Could you check a few things on this model? Use its own coordinates, in mm. Face numbers are marked on the shaded views. A direction names the side the tool comes from. Give positions to 0.01 mm unless a question says otherwise; leave off trailing zeros. Order: outer loops, then holes, each group sorted by start corner. A loop starts at its lowest first (then second) coordinate and runs counter-clockwise, first axis right, second up. Notation, with made-up numbers: (-28, 84) -> (-2, 84) arc R10 ccw to (-2, 88) -> close; hole circle Ø8 at (-13, -7). An arc over 180 degrees is marked (long way). Use one line per item in the form item = value. Start each with the question number.
from build123d import *

# Parameters (mm, degrees)
SKETCH6_R           = 23
BOSS_EXTRUDE3_DEPTH = 25
SKETCH7_R           = 1.5
CUT_EXTRUDE2_DEPTH  = 5
SKETCH8_R           = 1.25
CUT_EXTRUDE3_DEPTH  = 5
SKETCH9_R           = 4
BOSS_EXTRUDE4_DEPTH = 2
SKETCH10_R          = 2
BOSS_EXTRUDE5_DEPTH = 3
FILLET1_R           = 5
FILLET2_R           = 2
SKETCH11_W          = 63.139776453
SKETCH11_H          = 24.157827512
CUT_EXTRUDE4_DEPTH  = 50
SKETCH12_R          = 20
BOSS_EXTRUDE6_DEPTH = 5


with BuildPart() as part:
    # Sketch6 → Boss-Extrude3 (new body)
    with BuildSketch(Plane(origin=(0, 0, 0), x_dir=(1, 0, 0), z_dir=(0, 1, 0))):
        with Locations(Location((0, 0, 0), (0, 0, 270))):
            Circle(SKETCH6_R)
    extrude(amount=BOSS_EXTRUDE3_DEPTH)

    # Sketch7 → Cut-Extrude2 (cut)
    with BuildSketch(Plane(origin=(0, 0, 0), x_dir=(1, 0, 0), z_dir=(0, 1, 0))):
        with Locations(Location((-6, 0, 0), (0, 0, 270))):
            Circle(SKETCH7_R)
        with Locations(Location((0, 6, 0), (0, 0, 270))):
            Circle(SKETCH7_R)
        with Locations(Location((6, 0, 0), (0, 0, 270))):
            Circle(SKETCH7_R)
        with Locations(Location((0, -6, 0), (0, 0, 270))):
            Circle(SKETCH7_R)
    extrude(amount=CUT_EXTRUDE2_DEPTH, mode=Mode.SUBTRACT)

    # Sketch8 → Cut-Extrude3 (cut)
    with BuildSketch(Plane(origin=(0, 25, 0), x_dir=(1, 0, 0), z_dir=(0, 1, 0))):
        with Locations(Location((-13.856406461, -8, 0), (0, 0, 270))):
            Circle(SKETCH8_R)
        with Locations(Location((0, 16, 0), (0, 0, 270))):
            Circle(SKETCH8_R)
        with Locations(Location((13.856406461, -8, 0), (0, 0, 270))):
            Circle(SKETCH8_R)
    extrude(amount=-CUT_EXTRUDE3_DEPTH, mode=Mode.SUBTRACT)

    # Sketch9 → Boss-Extrude4 (add)
    with BuildSketch(Plane(origin=(0, 25, 0), x_dir=(1, 0, 0), z_dir=(0, 1, 0))):
        with Locations(Location((0, 0, 0), (0, 0, 270))):
            Circle(SKETCH9_R)
    extrude(amount=BOSS_EXTRUDE4_DEPTH)

    # Sketch10 → Boss-Extrude5 (add)
    with BuildSketch(Plane.XZ):
        with Locations(Location((0, 0, 0), (0, 0, 90))):
            Circle(SKETCH10_R)
    extrude(amount=BOSS_EXTRUDE5_DEPTH)

    # Fillet1
    fillet1_edges = [part.edges().sort_by_distance(p)[0] for p in [
        (0, 0, -23),
    ]]
    fillet(fillet1_edges, radius=FILLET1_R)

    # Fillet2
    fillet2_edges = [part.edges().sort_by_distance(p)[0] for p in [
        (0, 25, -23),
    ]]
    fillet(fillet2_edges, radius=FILLET2_R)

    # Sketch11 → Cut-Extrude4 (cut, symmetric)
    with BuildSketch(Plane(origin=(0, 0, 0), x_dir=(0, 0, -1), z_dir=(1, 0, 0))):
        with Locations((5.009304592, -2.078913756)):
            Rectangle(SKETCH11_W, SKETCH11_H)
    extrude(amount=CUT_EXTRUDE4_DEPTH, both=True, mode=Mode.SUBTRACT)

    # Sketch12 → Boss-Extrude6 (add)
    with BuildSketch(Plane.XZ.offset(-10)):
        with Locations(Location((0, 0, 0), (0, 0, 90))):
            Circle(SKETCH12_R)
    extrude(amount=BOSS_EXTRUDE6_DEPTH)


solid = part.part
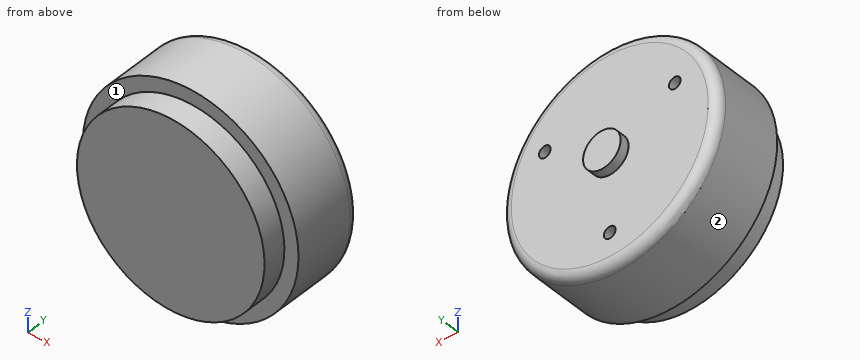
(1) Imagine slicing it at B-B (x = 0). Write out the boundary of the cut face in (y, z), plus the area to 3 significant figures.
(2) Imagine slicing it at C-C (y = 14). Write out the boundary of the cut face in (x, z).
(3) I'm going to push flat-ended pins straight in: pin 1 Ø4 at (y, z) = (18.5, -16.5) entering from +X; pin 2 Ø1.2 at (x, z) = (-0.5, -15.5) entering from +Y; pin 3 Ø21 at (x, z) = (-8, 7.5) entering from +Y; pin 4 Ø2 at (y, z) = (22.5, 0) entering from +X. Where does each tip first touch, or does it pass through?
(4) Which directions (+Z, -Z, +X, -X, +Y, -Y) give clear straight access to the entire face, cutting with the end or side of a thin tool? Please do the marked faces 1 and 2.
(5) Please list where these lines run through material, in increasing order: probe 1 along X at (y, z) = (24, 8); probe 2 along X at (y, z) = (23.3, 8); probe 3 along Y at (x, z) = (6, 19.5).
(6) Imagine slicing it at D-D (y = 21.5). Write out the boundary of the cut face in (x, z), plus the area to 3 significant figures.
(7) Imagine slicing it at A-A (z = 0). Write out the boundary of the cut face in (x, y).
Calculated:
q1.outline = (5, -20) -> (10, -20) -> (10, -23) -> (23, -23) arc R2 ccw to (25, -21) -> (25, -17.25) -> (20, -17.25) -> (20, -14.75) -> (25, -14.75) -> (25, -4) -> (27, -4) -> (27, 4) -> (25, 4) -> (25, 21) arc R2 ccw to (23, 23) -> (10, 23) -> (10, 20) -> (5, 20) -> close
q1.area = 892 mm2
q2.outline = circle Ø46 at (0, 0)
q3.pin_1 = 17.85
q3.pin_2 = 25
q3.pin_3 = 27
q3.pin_4 = 23
q4.face_1 = -Y
q4.face_2 = +Y, -Y
q5.probe_1 = -21.28 to -15.11, -12.61 to 12.61, 15.11 to 21.28
q5.probe_2 = -21.54 to -15.11, -12.61 to 12.61, 15.11 to 21.54
q5.probe_3 = 10 to 25
q6.outline = circle Ø46 at (0, 0); hole circle Ø2.5 at (-13.86, 8); hole circle Ø2.5 at (0, -16); hole circle Ø2.5 at (13.86, 8)
q6.area = 1,650 mm2
q7.outline = (-23, 10) -> (-20, 10) -> (-20, 5) -> (20, 5) -> (20, 10) -> (23, 10) -> (23, 23) arc R2 ccw to (21, 25) -> (4, 25) -> (4, 27) -> (-4, 27) -> (-4, 25) -> (-21, 25) arc R2 ccw to (-23, 23) -> close
